Model file for the job. Use its own axes, mm. A direction names the side the tool comes from. Coordinates: 2 decimals unless noted, no trailing zeros. Write each loop counter-clockwise with the first axis right and the second up, starting at its lowest first coordinate (ties: lowest second). Pieces come first, ordered by that corner, then holes. Notation, with made-up numbers: (0, 38.5) -> (49, 38.5) arc R27 ccw to (49, 57.5) -> close; hole circle Ø3 at (34, 50.25). An arc over 180 degrees is marked (long way). Answer as a JSON object with one key per item and string values. Group by question number.
from build123d import *

# Parameters (mm, degrees)
SKETCH2_R          = 3.25
CUT_EXTRUDE1_DEPTH = 10


with BuildPart() as part:
    # Sketch1 → Revolve1 (revolve)
    with BuildSketch(Plane.XY):
        Polygon((0, -4), (0, -14.5), (-20.063981043, -4), (-35, -4), (-35, 0), (-20, 0), (-20, 5.5), (-16, 5.5), (-16, -4), align=None)
    revolve(axis=Axis((0, 0, 0), (0, -1, 0)))

    # Sketch2 → Cut-Extrude1 (cut)
    with BuildSketch(Plane.XZ.offset(4)):
        with Locations((0, 28.5)):
            Circle(SKETCH2_R)
        with Locations((24.681724008, 14.25)):
            Circle(SKETCH2_R)
        with Locations((24.681724008, -14.25)):
            Circle(SKETCH2_R)
        with Locations((0, -28.5)):
            Circle(SKETCH2_R)
        with Locations((-24.681724008, -14.25)):
            Circle(SKETCH2_R)
        with Locations((-24.681724008, 14.25)):
            Circle(SKETCH2_R)
    extrude(amount=-CUT_EXTRUDE1_DEPTH, mode=Mode.SUBTRACT)


solid = part.part
(1) Cut at C-C on z = 14.25. Give the number of separate pieces and of enclosed holes in the cut face, plus the area to 3 significant figures.
(2) Wall check: probe 1 along Z at (x, y) = (0, -1.15); probe 2 along X at (y, z) = (-1.75, 12); probe 3 along Y at (x, z) = (-4, -25.5). Give the ranges that are in metal, low to high.
(3) Pull direction X, two halves, no side cores. Call faces 1 (the face through (0.27, -13.84, 1.23)), 2 (the face through (-0.705, -2.028, -31.673)), 3 (the face through (15, -4, 15)): released by +X, released by -X, zero draft, split by the parting line, or undercut.
(4) 3-axis set-ups, long thin cutter, end or side, ignore diameter. For faces 4 (the face through (3.47, 0.68, 15.62)), 5 (the face through (-21.582, -2.028, -13.274)): which of +Z, -Z, +X, -X, +Y, -Y reach the whole face in a straight line?
(5) Cut at D-D on x = 29.5. List the corners of the cut face in (y, z).
(6) Pin check, flat tips, straight feed: pin 1 (5 mm diameter, centred on x = -3, y = -11, fed in from -Z); pin 2 (10.5 mm diameter, centred on x = 24.68, z = -14.25, fed in from +Y); pin 3 (2 mm diameter, centred on y = -2.5, z = 25, fed in from +X). Stop position of each tip, or through.
(7) Cut at B-B on y = 4. List the corners of the cut face in (x, z).
(8) Cut at A-A on z = -28.5. List the corners of the cut face in (x, y), plus the area to 3 significant figures.
Results found:
{
 "1": {"separate pieces": "3", "enclosed holes": "0", "area": "275 mm²"},
 "2": {"probe 1": "z = -35 to -31.75, -25.25 to -16, 16 to 25.25, 31.75 to 35", "probe 2": "x = -32.88 to -27.03, -22.34 to -10.58, 10.58 to 22.34, 27.03 to 32.88", "probe 3": "y = -4 to 0"},
 "3": {"face 1": "split by the parting line", "face 2": "undercut", "face 3": "zero draft"},
 "4": {"face 4": "+Y", "face 5": "+Y, -Y"},
 "5": {"outline": "(-4, -18.83) -> (0, -18.83) -> (0, 18.83) -> (-4, 18.83) -> close"},
 "6": {"pin 1": "stops at z = -11.11", "pin 2": "stops at y = 0", "pin 3": "stops at x = 25.48"},
 "7": {"outline": "circle Ø40 at (0, 0); hole circle Ø32 at (0, 0)"},
 "8": {"outline": "(-20.32, -4) -> (-3.25, -4) -> (-3.25, 0) -> (-20.32, 0) -> close; (3.25, -4) -> (20.32, -4) -> (20.32, 0) -> (3.25, 0) -> close", "area": "137 mm²"}
}
